Part print with two shaded views. Sizes in mm from the minimum x, y, z corner. Give positions to 0.01 mm unless a question says otherwise; leave off trailing zeros. Order: outer loops, then holes, each group sorted by start corner. A loop starts at its lowest first (then second) coordinate and runs counter-clockwise, first axis right, second up.
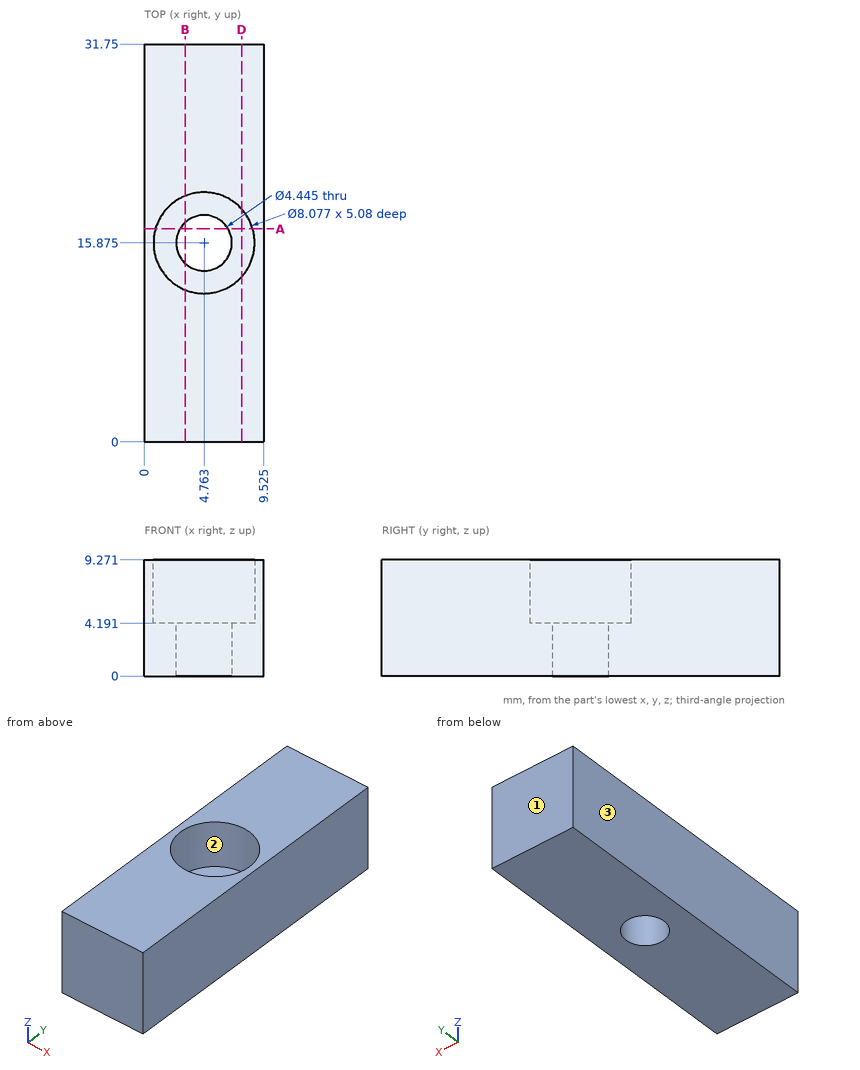
Item 1: Slice it at A-A (y = 17). Give the cut face in (x, z) (1 decimal).
Item 2: Slice it at D-D (x = 7.75). Give the cut face in (y, z), and give its area (3 significant figures).
Item 3: Slice it at B-B (x = 3.25). Give the cut face in (y, z), and give its area (3 significant figures).
Item 4: Wall check: L1, parallel to Z at x = 6.5, y = 19; L2, parallel to Y at x = 2, z = 7; L3, parallel to X at y = 18, z = 7.25 (1 decimal). Give the ranges that are in metal, low to high.
Item 5: Two-plate mould, pull along X, no slides. Class the marked faces 1, 2 and 3: released by +X, released by -X, zero draft, split by the parting line, or undercut.
A:
1. outline: (0, 0) - (2.8, 0) - (2.8, 4.2) - (0.9, 4.2) - (0.9, 9.3) - (0, 9.3) - close; (6.7, 0) - (9.5, 0) - (9.5, 9.3) - (8.6, 9.3) - (8.6, 4.2) - (6.7, 4.2) - close
2. outline: (0, 0) - (31.75, 0) - (31.75, 9.27) - (18.59, 9.27) - (18.59, 4.19) - (13.16, 4.19) - (13.16, 9.27) - (0, 9.27) - close
2. area: 267 mm2
3. outline: (0, 0) - (14.25, 0) - (14.25, 4.19) - (12.13, 4.19) - (12.13, 9.27) - (0, 9.27) - close; (17.5, 0) - (31.75, 0) - (31.75, 9.27) - (19.62, 9.27) - (19.62, 4.19) - (17.5, 4.19) - close
3. area: 243 mm2
4. L1: z = 0 to 4.19
4. L2: y = 0 to 12.93, 18.82 to 31.75
4. L3: x = 0 to 1.3, 8.2 to 9.5
5. face 1: zero draft
5. face 2: undercut
5. face 3: released by -X
